Read the model definition and answer for the solid it produces. Units are mm, in the model's axes. A direction names the side the tool comes from. Round coordinates to 2 decimals unless told otherwise and drop trailing zeros. Order: outer loops, then holes, each group sorted by start corner. A loop starts at its lowest first (then second) coordinate and runs counter-clockwise, first axis right, second up. Notation, with made-up numbers: (28, -12) - (38, -12) arc R14 cw to (38, -8) - close; hole circle Ø1 at (45.5, 10). An arc over 180 degrees is marked (long way). Answer as a JSON object with one key per item and string values. Group by question number.
Q1. Given pin 1 Ø3 at (x, z) = (6, 96.5) entering from -Y; pin 2 Ø0.6 at (x, y) = (-0.5, -36) entering from +Z; pin 3 Ø8 at (y, z) = (-85, 103.5) entering from +X; pin 4 Ø1 at (x, y) = (0.5, -35.5) entering from -Z, each flat-ended and moving along its own axis, determine where each tip first touches the part or whether it passes through.
Q2. Consider line 1 (Y direction, x = 6, z = 99.25); line 2 (X direction, y = -65.5, z = 101); line 3 (Z direction, x = 0.75, y = -98.5). Determine where each line is inside the solid, lowest interval first.
Q3. A cutting plane is placed at A-A on x = 0. Determine the outline of the cut face in (y, z), and give its area (4 significant figures).
Q4. A cutting plane is placed at B-B on y = -89. Determine the outline of the cut face in (x, z), and give its area (3 significant figures).
Q5. The mould has two halves that part along Z. Classify faces 4 (the flat face through (0.1, -37, 97.8)), 5 (the flat face through (0, -35, 103)), 6 (the cylindrical face through (1.63, -36.26, 93.68)): pulls with the +Z half, pulls with the -Z half, needs draft (parallel to the pull), parting line crosses it, or undercut.
Q6. A tool of negligible diameter and unlimited length cuts with its end or side. For faces 1 (the flat face through (1.74, -35.49, 100.01)), 2 (the flat face through (0, -107, 101)), 3 (the cylindrical face through (0.65, -71.51, 103.93)), from which of +Z, -Z, +X, -X, +Y, -Y can it reach the whole face along a straight path? Write none if from no direction.
```python
from build123d import *

# Parameters (mm, degrees)
SKETCH090_R             = 7.5
PAD060_DEPTH            = 2.5
CHAMFER_SIZE            = 1
POCKET022_DEPTH         = 2
SKETCH092_R             = 3
PAD061_DEPTH            = 70
BODY051_PLACEMENT_ANGLE = 90
BODY052_PLACEMENT_ANGLE = 180


with BuildPart() as part:
    # Sketch090 → Pad060 (new body)
    with BuildSketch(Plane.XY):
        Circle(SKETCH090_R)
    extrude(amount=PAD060_DEPTH)

    # Chamfer
    chamfer_edges = [part.edges().sort_by_distance(p)[0] for p in [
        (-7.5, 0, 2.5),
    ]]
    chamfer(chamfer_edges, length=CHAMFER_SIZE)

    # Sketch091 (on Face4 of Chamfer) → Pocket022 (cut)
    with BuildSketch(Plane.XY.offset(2.5)):
        Polygon((1.154701, 2), (-1.154701, 2), (-2.309401, 0), (-1.154701, -2), (1.154701, -2), (2.309401, 0), align=None)
    extrude(amount=-POCKET022_DEPTH, mode=Mode.SUBTRACT)

    # Sketch092 (on Face3 of Pocket022) → Pad061 (join)
    with BuildSketch(Plane(origin=(0, 0, 0), x_dir=(1, 0, 0), z_dir=(0, 0, -1))):
        Circle(SKETCH092_R)
    extrude(amount=PAD061_DEPTH)


with BuildPart() as part_1:
    # Body051 placement: moved
    add(part.part.moved(Location((0, 37, 101))).rotate(Axis((0, 37, 101), (1, 0, 0)), BODY051_PLACEMENT_ANGLE))


with BuildPart() as part_2:
    # Body052 placement: moved
    add(part_1.part.rotate(Axis((0, 0, 0), (0, 0, 1)), BODY052_PLACEMENT_ANGLE))


solid = part_2.part
```
Result set:
{
 "1": {"pin 1": "stops at y = -37", "pin 2": "stops at z = 108.5", "pin 3": "stops at x = 3", "pin 4": "stops at z = 93.5"},
 "2": {"line 1": "y = -37 to -34.5", "line 2": "x = -3 to 3", "line 3": "z = 98.1 to 103.9"},
 "3": {"outline": "(-107, 98) - (-37, 98) - (-37, 93.5) - (-35.5, 93.5) - (-34.5, 94.5) - (-34.5, 99) - (-36.5, 99) - (-36.5, 103) - (-34.5, 103) - (-34.5, 107.5) - (-35.5, 108.5) - (-37, 108.5) - (-37, 104) - (-107, 104) - close", "area": "448.5 mm²"},
 "4": {"outline": "circle Ø6 at (0, 101)", "area": "28.3 mm²"},
 "5": {"face 4": "needs draft", "face 5": "undercut", "face 6": "parting line crosses it"},
 "6": {"face 1": "+Y", "face 2": "+Z, -Z, +X, -X, -Y", "face 3": "-Y"}
}
